```python
from build123d import *

# Parameters (mm, degrees)
F0_W     = 31.75
F0_H     = 73.025
F1_DEPTH = 31.75
F2_R     = 15.875
F2_R_2   = 12.954
F3_DEPTH = 17.78
F4_DEPTH = 31.751
F5_DEPTH = 31.751
F6_DEPTH = 29.21
F7_R     = 12.954
F8_DEPTH = 57.15


with BuildPart() as f1:
    # F0 (on Top) → F1 (new body)
    with BuildSketch(Plane.XY):
        Rectangle(F0_W, F0_H)
    extrude(amount=F1_DEPTH)

    # F2 (on face) → F3 (join)
    with BuildSketch(Plane.XY.offset(31.75)):
        with Locations((0, 20.6375)):
            Circle(F2_R)
        with Locations((0, 20.6375)):
            Circle(F2_R_2, mode=Mode.SUBTRACT)
    extrude(amount=F3_DEPTH)

    # F4 (cut, through all): a face of the model
    f4_faces = [f1.faces().sort_by_distance(p)[0] for p in [
        (-12.3290339692, 32.9665339692, 31.75),
    ]]
    extrude(f4_faces, amount=-F4_DEPTH, mode=Mode.SUBTRACT)

    # F5 (cut, through all): a face of the model
    f5_faces = [f1.faces().sort_by_distance(p)[0] for p in [
        (12.3290339692, 32.9665339692, 31.75),
    ]]
    extrude(f5_faces, amount=-F5_DEPTH, mode=Mode.SUBTRACT)

    # F6 (cut): a face of the model
    f6_faces = [f1.faces().sort_by_distance(p)[0] for p in [
        (0, 20.6375, 31.75),
    ]]
    extrude(f6_faces, amount=-F6_DEPTH, mode=Mode.SUBTRACT)

    # F7 (on face) → F8 (cut)
    with BuildSketch(Plane.XZ.offset(36.5125)):
        with Locations((0, 15.875)):
            Circle(F7_R)
    extrude(amount=-F8_DEPTH, mode=Mode.SUBTRACT)


solid = f1.part
```
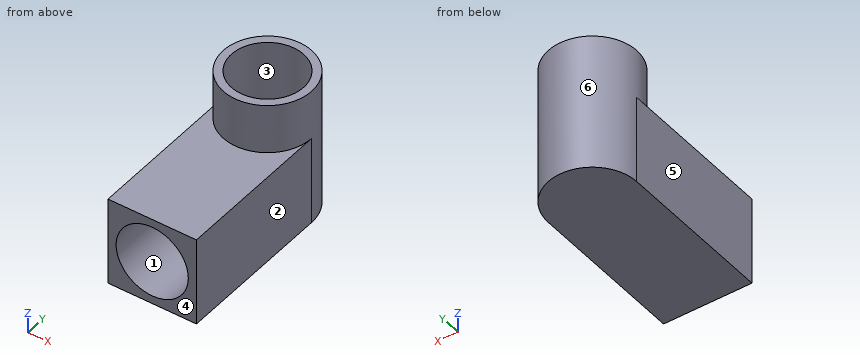
Build history of the part. All positions in model axes, mm. Face numbers are marked on the shaded views. A direction names the side the tool comes from. Give positions to 0.01 mm unless a question says otherwise; leave off trailing zeros. Loops run counter-clockwise (first coordinate to the right, second up) from the corner with the lowest first, then second, coordinate; pieces in that order, holes last. Notation, with made-up numbers: (-38, -7) - (17, -7) arc R27 ccw to (17, 22) - close; hole circle Ø11 at (40, -27.75). An arc over 180 degrees is marked (long way). Use a Markdown table: item, result.
(1) Pull direction Y, two halves, no side cores. Call the marked faces 3, 4, 5 and 6: +Y half, -Y half, draft (parallel to the pull), parting line (faces both ways), or undercut.
Taken from the geometry:
| item | result |
|---|---|
| face 3 | undercut |
| face 4 | -Y half |
| face 5 | draft |
| face 6 | parting line |
(2) Band-saw the part on B-B (y = -4.5). Give the cut face in (x, z) (3 decimals), and give its area (3 significant figures).
Taken from the geometry:
| item | result |
|---|---|
| outline | (-15.875, 0) - (15.875, 0) - (15.875, 31.75) - (-15.875, 31.75) - close; hole circle Ø25.908 at (0, 15.875) |
| area | 481 mm2 |
(3) Band-saw the part on A-A (x = 0). Give the cut face in (y, z).
Taken from the geometry:
| item | result |
|---|---|
| outline | (-36.51, 0) - (36.51, 0) - (36.51, 49.53) - (33.59, 49.53) - (33.59, 2.54) - (7.68, 2.54) - (7.68, 2.92) - (-36.51, 2.92) - close; (-36.51, 28.83) - (7.68, 28.83) - (7.68, 49.53) - (4.76, 49.53) - (4.76, 31.75) - (-36.51, 31.75) - close |
(4) Which spindle directions (+Z, -Z, +X, -X, +Y, -Y) get a long thin tool onto all of the face, cutting with end or side? Do the marked faces 1 and 2. Say none if no direction does.
Taken from the geometry:
| item | result |
|---|---|
| face 1 | -Y |
| face 2 | +Z, -Z, +X, +Y, -Y |
(5) Drop flat-ended pins along their axis: pin 1 Ø1.5 at (y, z) = (23, 23.5) entering from +X; pin 2 Ø1 at (x, z) = (-1.5, 17.5) entering from -Y; pin 3 Ø16 at (x, y) = (2.5, -16.5) entering from +Z. Give the stop position or say it passes through.
Taken from the geometry:
| item | result |
|---|---|
| pin 1 | x = 15.79 |
| pin 2 | y = 33.44 |
| pin 3 | z = 31.75 |
(6) Wall check: line 1 along Z through (x, y) = (0, 2); line 2 along Y through (x, z) = (0, 42.5); line 3 along Y through (x, z) = (10, 4). Give the ranges that are in metal, low to high.
Taken from the geometry:
| item | result |
|---|---|
| line 1 | 0 to 2.92, 28.83 to 31.75 |
| line 2 | 4.76 to 7.68, 33.59 to 36.51 |
| line 3 | -36.51 to 12.4, 28.87 to 32.97 |
